CAD build for the part. Positions are in the model's coordinates, mm. Face numbers are marked on the shaded views. A direction names the side the tool comes from. Coordinates: 2 decimals unless noted, no trailing zeros. Loops run counter-clockwise (first coordinate to the right, second up) from the corner with the lowest first, then second, coordinate; pieces in that order, holes last.
1) Wall check: line 1 along Y through (x, z) = (-1, 19); line 2 along Y through (x, z) = (-4, 0.85). Give the ranges that are in metal, low to high.
2) Which spindle directions (+Z, -Z, +X, -X, +Y, -Y) get a long thin tool onto all of the face, cutting with end or side? Do the marked faces 1 and 2. Say none if no direction does.
3) Pin check, flat tips, straight feed: pin 1 Ø3 at (x, z) = (-2, 32.5) entering from -Y; pin 2 Ø4 at (x, z) = (-6, 35) entering from +Y; pin 3 Ø4 at (x, y) = (-1.5, 4.5) entering from +Z; pin 4 Ø2.5 at (x, y) = (-3, 9.5) entering from +Z. Stop position of each tip, or through.
4) Saw through at B-B, the plane x = -7. Write the cut outline in (y, z).
5) Saw through at A-A, the plane y = 10. Write the cut outline in (x, z), and give its area (3 significant figures).
6) Saw through at C-C, the plane z = 5.5. Write the cut outline in (x, y).
```python
from build123d import *

# Parameters (mm, degrees)
F2_W     = 8
F2_H     = 1
F5_D     = 3.3
F7_D     = 3.3
F9_DEPTH = 15.001


with BuildPart() as f3:
    # F3: sweep along a path in F0
    with BuildLine(Plane.YZ) as f3_path:
        Line((15, 0), (5, 0))
        ThreePointArc((5, 0), (1.4644660941, 1.4644660941), (0, 5))
        Line((0, 5), (0, 50.8934259415))
    # F2 (on line) → F3 (sweep)
    with BuildSketch(Plane.XZ.offset(-15)):
        with Locations((-4, 0.5)):
            Rectangle(F2_W, F2_H)
    sweep(path=f3_path.line)

    # F5 (through all)
    with Locations(Plane.XY.offset(1)):
        with Locations((-4, 10)):
            Hole(F5_D / 2)

    # F7 (through all)
    with Locations(Plane.XZ):
        with Locations((-4, 47.1934259415)):
            Hole(F7_D / 2)

    # F8 (on face) → F9 (cut, through all)
    with BuildSketch(Plane.XZ):
        with BuildLine():
            add(Edge.make_bspline(
                [(0, 47.1934259415), (0, 50.8934259415), (-4, 50.8934259415)],
                knots=[0, 0, 0, 1.5707963268, 1.5707963268, 1.5707963268], degree=2, weights=[1, 0.7071067812, 1]))
            Line((0, 47.1934259415), (0, 50.8934259415))
            Line((0, 50.8934259415), (-4, 50.8934259415))
        make_face()
    extrude(amount=-F9_DEPTH, mode=Mode.SUBTRACT)


solid = f3.part
```
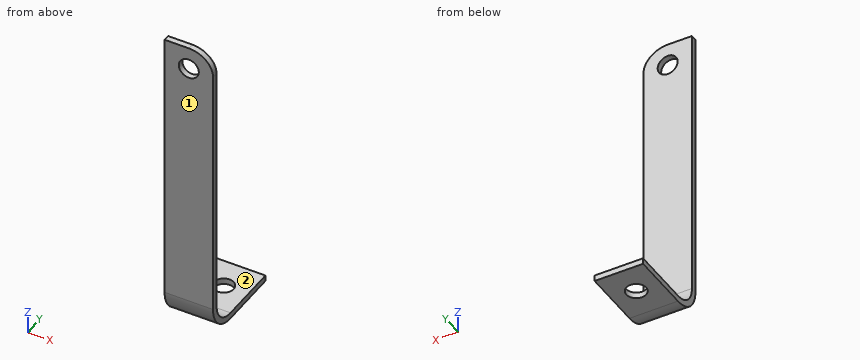
Data:
1. line 1: y = 0 to 1
1. line 2: y = 2.21 to 8.35, 11.65 to 15
2. face 1: +Z, -Z, +X, -X, -Y
2. face 2: +Z, +X, -X, +Y
3. pin 1: stops at y = 0
3. pin 2: stops at y = 1
3. pin 3: stops at z = 1.88
3. pin 4: stops at z = 1
4. outline: (0, 5) arc R5 ccw to (5, 0) - (15, 0) - (15, 1) - (5, 1) arc R4 cw to (1, 5) - (1, 50.89) - (0, 50.89) - close
5. outline: (-8, 0) - (-5.65, 0) - (-5.65, 1) - (-8, 1) - close; (-2.35, 0) - (0, 0) - (0, 1) - (-2.35, 1) - close
5. area: 4.70 mm2
6. outline: (-8, 0) - (0, 0) - (0, 1) - (-8, 1) - close
